from build123d import *
from OCP.BRepAlgoAPI import BRepAlgoAPI_Cut
from OCP.TopTools import TopTools_ListOfShape

# Parameters (mm, degrees)
SKETCH1_R              = 3
BOSS_EXTRUDE1_DEPTH    = 28.575
CUT_EXTRUDE1_DEPTH     = 18.034
CUT_EXTRUDE4_DEPTH     = 6.35
CUT_EXTRUDE5_START     = -28.575
CUT_EXTRUDE5_OUTLINE_R = 4
CUT_EXTRUDE5_DEPTH     = 28.575


with BuildPart() as part:
    # Sketch1 → Boss-Extrude1 (new body)
    with BuildSketch(Plane(origin=(0, 0, 0), x_dir=(1, 0, 0), z_dir=(0, 1, 0))):
        Polygon((0, 6.35), (0, 22.225), (0, 28.575), (6.35, 28.575), (57.15, 28.575), (63.5, 28.575), (63.5, 22.225), (63.5, 6.35), (63.5, 0), (57.15, 0), (6.35, 0), (0, 0), align=None)
        with Locations(Location((12.7, 14.2875, 0), (0, 0, 270))):
            Circle(SKETCH1_R, mode=Mode.SUBTRACT)
        with Locations(Location((50.8, 14.2875, 0), (0, 0, 270))):
            Circle(SKETCH1_R, mode=Mode.SUBTRACT)
    extrude(amount=-BOSS_EXTRUDE1_DEPTH)

    # Sketch2 → Cut-Extrude1 (cut)
    with BuildSketch(Plane(origin=(0, 0, 0), x_dir=(1, 0, 0), z_dir=(0, 1, 0))):
        with BuildLine():
            Line((6.985, 24.765), (56.515, 24.765))
            ThreePointArc((56.515, 24.765), (58.76006403, 23.83506403), (59.69, 21.59))
            Line((59.69, 21.59), (59.69, 6.985))
            ThreePointArc((59.69, 6.985), (58.76006403, 4.73993597), (56.515, 3.81))
            Line((56.515, 3.81), (6.985, 3.81))
            ThreePointArc((6.985, 3.81), (4.73993597, 4.73993597), (3.81, 6.985))
            Line((3.81, 6.985), (3.81, 21.59))
            ThreePointArc((3.81, 21.59), (4.73993597, 23.83506403), (6.985, 24.765))
        make_face()
    extrude(amount=-CUT_EXTRUDE1_DEPTH, mode=Mode.SUBTRACT)

    # Sketch4 → Cut-Extrude4 (cut)
    with BuildSketch(Plane(origin=(0, -18.034, 0), x_dir=(1, 0, 0), z_dir=(0, 1, 0))):
        with BuildLine():
            Line((55.850907282, 18.135984848), (52.706002748, 22.263484848))
            ThreePointArc((52.706002748, 22.263484848), (50.473305999, 24.105359338), (47.655095466, 24.765))
            Line((47.655095466, 24.765), (15.844904534, 24.765))
            ThreePointArc((15.844904534, 24.765), (13.026694001, 24.105359338), (10.793997252, 22.263484848))
            Line((10.793997252, 22.263484848), (7.649092718, 18.135984848))
            ThreePointArc((7.649092718, 18.135984848), (6.35, 14.2875), (7.649092718, 10.439015152))
            Line((7.649092718, 10.439015152), (10.793997252, 6.311515152))
            ThreePointArc((10.793997252, 6.311515152), (13.026694001, 4.469640662), (15.844904534, 3.81))
            Line((15.844904534, 3.81), (47.655095466, 3.81))
            ThreePointArc((47.655095466, 3.81), (50.473305999, 4.469640662), (52.706002748, 6.311515152))
            Line((52.706002748, 6.311515152), (55.850907282, 10.439015152))
            ThreePointArc((55.850907282, 10.439015152), (57.15, 14.2875), (55.850907282, 18.135984848))
        make_face()
    extrude(amount=-CUT_EXTRUDE4_DEPTH, mode=Mode.SUBTRACT)


with BuildPart() as cut_extrude5_tool:
    # Cut-Extrude5: read off the stored shape, not the designer's step
    # Cut-Extrude5 outline → Cut-Extrude5 (new body)
    with BuildSketch(Plane(origin=(0, 0, -28.575), x_dir=(-1, 0, 0), z_dir=(0, 0, -1)).offset(CUT_EXTRUDE5_START)):
        with BuildLine():
            ThreePointArc((-31.75, 4.067e-06), (-29.462231849, -0.278821364), (-27.308403366, -1.098973545))
            Line((-27.308403366, -1.098973545), (-1.694470317, -14.600801413))
            ThreePointArc((-1.694470317, -14.600801413), (-0.456425728, -15.769363319), (-1.896e-06, -17.409475699))
            Line((-1.896e-06, -17.409475699), (0, 0))
            Line((0, 0), (-31.75, 4.067e-06))
        make_face()
        with BuildLine():
            ThreePointArc((-36.191594414, -1.098972375), (-34.037766933, -0.278821063), (-31.75, 4.067e-06))
            Line((-31.75, 4.067e-06), (-63.5, 0))
            Line((-63.5, 0), (-63.500001896, -17.409469074))
            ThreePointArc((-63.500001896, -17.409469074), (-63.043577848, -15.769356336), (-61.805532735, -14.600794399))
            Line((-61.805532735, -14.600794399), (-36.191594414, -1.098972375))
        make_face()
        with BuildLine():
            Line((0, -28.575), (-1.896e-06, -25.399996402))
            ThreePointArc((-1.896e-06, -25.399996402), (-0.929937865, -27.645060432), (-3.175001896, -28.574996402))
            Line((-3.175001896, -28.574996402), (0, -28.575))
        make_face()
        with BuildLine():
            ThreePointArc((-60.325001896, -28.574996402), (-62.570065927, -27.645060433), (-63.500001896, -25.399996402))
            Line((-63.500001896, -25.399996402), (-63.5, -28.575))
            Line((-63.5, -28.575), (-60.325001896, -28.574996402))
        make_face()
        with Locations((-31.75, -9.525)):
            Circle(CUT_EXTRUDE5_OUTLINE_R)
    extrude(amount=CUT_EXTRUDE5_DEPTH)


with BuildPart() as part_1:
    add(part.part)

    # Cut-Extrude5: cut by cut_extrude5_tool, with a tolerance
    cut_extrude5_stock = TopTools_ListOfShape()
    cut_extrude5_stock.Append(part_1.part.wrapped)
    cut_extrude5_tools = TopTools_ListOfShape()
    cut_extrude5_tools.Append(cut_extrude5_tool.part.wrapped)
    cut_extrude5_cut = BRepAlgoAPI_Cut()
    cut_extrude5_cut.SetArguments(cut_extrude5_stock)
    cut_extrude5_cut.SetTools(cut_extrude5_tools)
    cut_extrude5_cut.SetFuzzyValue(0.00001)
    cut_extrude5_cut.Build()
    add(Compound.cast(cut_extrude5_cut.Shape()).solids(), mode=Mode.REPLACE)


solid = part_1.part
Geometry check sheet. Reference: the model listing, model coordinates, mm. A direction names the side the tool comes from. Round coordinates to 2 decimals unless told otherwise and drop trailing zeros. Order: outer loops, then holes, each group sorted by start corner. A loop starts at its lowest first (then second) coordinate and runs counter-clockwise, first axis right, second up. Notation, with made-up numbers: M 54,-22 L 100,-22 A37 ccw 100,16 Z; hole C 80,-29 d9. An arc over 180 degrees is marked long. Answer in a Markdown table with one row per item. Add a question column.
Item 1: Set-up check for faces 1 (the face through (12.99, -21.16, -4.49)), 2 (the face through (34.924, -11.959, -1.878)): record each of +Z, -Z, +X, -X, +Y, -Y from which the full face is reachable in a straight line by a thin tool's end or side.
Item 2: Depth check by flat-ended pin: pin 1 Ø3.5 at (x, z) = (10, -14) entering from +Y; pin 2 Ø3 at (x, z) = (52.5, -4) entering from +Y; pin 3 Ø12 at (y, z) = (-7.5, -6) entering from -X. Enter the tip coordinate at first touch or a pass-through.
Item 3: Draft check along X on faces 3 (the face through (62.545, -27.67, -14.087)), 4 (the face through (4.76, -15.57, -4.72)), 5 (the face through (32, -28.575, -14)). Enter one of: released by +X, released by -X, zero draft, split by the parting line, or undercut.
Item 4: Material ranges on L1, parallel to Y at x = 31.75, z = -1.45 (3 decimals); L2, parallel to Z at x = 43, y = -8.5 (3 decimals); L3, parallel to X at y = -17.25, z = -14, recorded low to high. Write a range as [from, to].
Item 5: Sectioned sample at B-B, the plane x = 50.8. Enter the section's corners in (y, z) (1 decimal).
Item 6: Sectioned sample at C-C, the plane z = -15.25. Enter the section's corners in (x, y) (3 decimals).
Item 7: Sectioned sample at D-D, the plane y = -6.25. Enter the section's corners in (x, z) (3 decimals), plus the area to 3 significant figures.
Filled in:
| question | item | result |
|---|---|---|
| 1 | face 1 | +Y |
| 1 | face 2 | +Z, -Z |
| 2 | pin 1 | stops at y = -24.38 |
| 2 | pin 2 | stops at y = -8.91 |
| 2 | pin 3 | stops at x = 3.78 |
| 3 | face 3 | released by +X |
| 3 | face 4 | undercut |
| 3 | face 5 | zero draft |
| 4 | L1 | y = [-28.575, -13.525], [-5.525, 0] |
| 4 | L2 | z = [-28.575, -24.765], [-3.81, 0] |
| 4 | L3 | x = [0, 3.81], [59.69, 63.5] |
| 5 | outline | M -28.6,-28.6 L -8.8,-28.6 L -8.8,-24.8 L -18,-24.8 L -18,-23.9 L -24.4,-23.9 L -24.4,-17.3 L -28.6,-17.3 Z; M -28.6,-11.3 L -24.4,-11.3 L -24.4,-4.6 L -18,-4.6 L -18,-3.8 L -8.8,-3.8 L -8.8,0 L -28.6,0 Z |
| 6 | outline | M 0,-25.4 A3.175 ccw 3.175,-28.575 L 9.859,-28.575 L 9.859,-24.384 L 6.423,-24.384 L 6.423,-18.034 L 3.81,-18.034 L 3.81,-13.486 L 1.694,-14.601 A3.175 ccw 0,-17.409 Z; M 15.541,-28.575 L 47.959,-28.575 L 47.959,-24.384 L 15.541,-24.384 Z; M 53.641,-28.575 L 60.325,-28.575 A3.175 ccw 63.5,-25.4 L 63.5,-17.409 A3.175 ccw 61.806,-14.601 L 59.69,-13.486 L 59.69,-18.034 L 57.077,-18.034 L 57.077,-24.384 L 53.641,-24.384 Z |
| 7 | outline | M 17.537,-28.575 L 29.453,-28.575 L 29.453,-24.765 L 17.537,-24.765 Z; M 17.537,-3.81 L 29.453,-3.81 L 29.453,0 L 17.537,0 Z; M 34.047,-28.575 L 45.963,-28.575 L 45.963,-24.765 L 34.047,-24.765 Z; M 34.047,-3.81 L 45.963,-3.81 L 45.963,0 L 34.047,0 Z |
| 7 | area | 182 mm² |
